Geometry: see drawing. Coordinates: mm, zero at the bounding-box minimum. A direction names the side the tool comes from. Give positions to 0.01 mm unless a question says otherwise; leave off trailing zeros. Order: outer loops, then holes, each group sorted by start corner. A loop starts at its lowest first (then second) coordinate and runs counter-clockwise, first axis right, second up. Notation, with made-up numbers: (-27, 23) - (-22, 23) arc R15 cw to (-22, 41) - close; hole circle Ø4 at (-24.5, 10.5). An arc over 180 degrees is marked (long way). One line per item, written item: value.
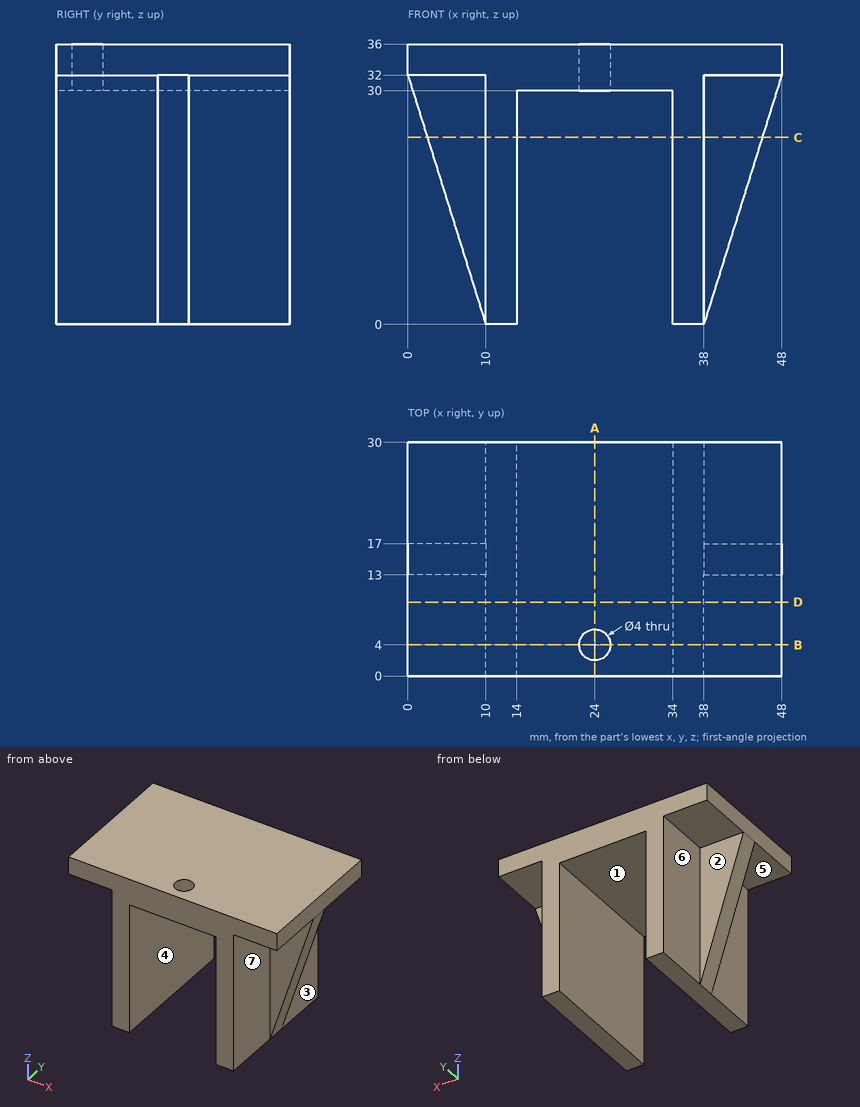
1) Section C-C, the plane z = 24. Return loops of the section in (x, y), then the cut area to 3 significant figures.
Answers below:
outline: (2.5, 13) - (10, 13) - (10, 0) - (14, 0) - (14, 30) - (10, 30) - (10, 17) - (2.5, 17) - close; (34, 0) - (38, 0) - (38, 13) - (45.5, 13) - (45.5, 17) - (38, 17) - (38, 30) - (34, 30) - close
area: 300 mm^2
2) Material intervals for line 1 along X through (y, z) = (20.5, 26); line 2 along Y through (x, z) = (24, 33.45); line 3 along Z through (x, y) = (24, 12), sorted ascending.
Answers below:
line 1: 10 to 14, 34 to 38
line 2: 0 to 2, 6 to 30
line 3: 30 to 36
3) Mould query, pull axis X, two halves, no side actions, for the marked faces 1, 2 and 3. Classes: released by +X, released by -X, zero draft, split by the parting line, or undercut.
Answers below:
face 1: undercut
face 2: zero draft
face 3: released by +X
4) First-contact query: pin 1 (4 mm diameter, centred on y = 6.5, z = 23.5, fed in from -X); pin 2 (4 mm diameter, centred on y = 4.5, z = 16.5, fed in from +X); pin 3 (9 mm diameter, centred on y = 13.5, z = 19.5, fed in from +X). Flat tips, straight axial feed; report the tip coordinate or a pass-through.
Answers below:
pin 1: x = 10
pin 2: x = 38
pin 3: x = 45.5
5) Section B-B, the plane y = 4. Return loops of the section in (x, z), then the cut area to 3 significant figures.
Answers below:
outline: (0, 32) - (10, 32) - (10, 0) - (14, 0) - (14, 30) - (22, 30) - (22, 36) - (0, 36) - close; (26, 30) - (34, 30) - (34, 0) - (38, 0) - (38, 32) - (48, 32) - (48, 36) - (26, 36) - close
area: 464 mm^2
6) Section D-D, the plane y = 9.5. Return loops of the section in (x, z).
Answers below:
outline: (0, 32) - (10, 32) - (10, 0) - (14, 0) - (14, 30) - (34, 30) - (34, 0) - (38, 0) - (38, 32) - (48, 32) - (48, 36) - (0, 36) - close
7) Set-up query: the marked faces 4, 5, 6 and 7. Return all of +Z, -Z, +X, -X, +Y, -Y with unobstructed straight access to the full face (end or side cutting, diameter ignored); none if empty.
Answers below:
face 4: -Z, +Y, -Y
face 5: -Z, -X, -Y
face 6: -Z, -X, +Y
face 7: -Z, +X, -Y
8) Section A-A, the plane x = 24. Return loops of the section in (y, z).
Answers below:
outline: (0, 30) - (2, 30) - (2, 36) - (0, 36) - close; (6, 30) - (30, 30) - (30, 36) - (6, 36) - close
